Here's how the part is built. I have some questions about the finished solid (model axes, mm). Face numbers are marked on the shaded views. A direction names the side the tool comes from. Round coordinates to 2 decimals unless told otherwise and drop trailing zeros. Loops run counter-clockwise (first coordinate to the right, second up) from the corner with the lowest first, then second, coordinate; pieces in that order, holes last. Notation, with made-up numbers: M 42,-23 L 53,-23 A23 ccw 53,5 Z; hole C 38,-6 d5. An arc over 180 degrees is marked long. Write each question's results on one line, items separated by ' | '. Start each with the question number.
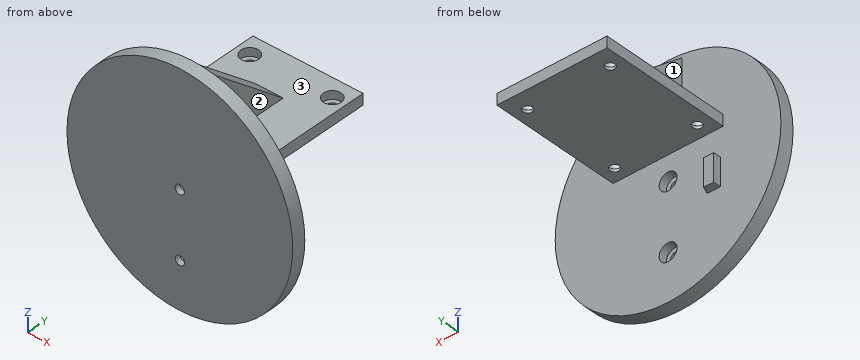
```python
from build123d import *

# Parameters (mm, degrees)
SKETCH1_R                                    = 41
BOSS_EXTRUDE1_DEPTH                          = 5
BOSS_EXTRUDE2_DEPTH                          = 5.08
BOSS_EXTRUDE2_DEPTH_BACK                     = 5.08
SKETCH7_W                                    = 40
SKETCH7_H                                    = 48
BOSS_EXTRUDE3_DEPTH                          = 4
CBORE_FOR_M5_HEX_HEAD_CAP_SCREW5_D           = 3.4
CBORE_FOR_M5_HEX_HEAD_CAP_SCREW5_DEPTH       = 5.5
CBORE_FOR_M5_HEX_HEAD_CAP_SCREW5_CBORE_D     = 6.5
CBORE_FOR_M5_HEX_HEAD_CAP_SCREW5_CBORE_DEPTH = 3
CBORE_FOR_M5_HEX_HEAD_CAP_SCREW5_TIP         = 1.021463052
SKETCH22_W                                   = 4
SKETCH22_H                                   = 10
BOSS_EXTRUDE4_DEPTH                          = 2
BOSS_EXTRUDE5_DEPTH                          = 10
CBORE_FOR_M5_HEX_HEAD_CAP_SCREW6_D           = 3.4
CBORE_FOR_M5_HEX_HEAD_CAP_SCREW6_DEPTH       = 5.5
CBORE_FOR_M5_HEX_HEAD_CAP_SCREW6_CBORE_D     = 6.5
CBORE_FOR_M5_HEX_HEAD_CAP_SCREW6_CBORE_DEPTH = 3
CBORE_FOR_M5_HEX_HEAD_CAP_SCREW6_TIP         = 1.021463052


with BuildPart() as part:
    # Sketch1 → Boss-Extrude1 (new body)
    with BuildSketch(Plane(origin=(0, 0, 0), x_dir=(1, 0, 0), z_dir=(0, 1, 0))):
        with Locations(Location((0, 0, 0), (0, 0, 270))):
            Circle(SKETCH1_R)
    extrude(amount=BOSS_EXTRUDE1_DEPTH)

    # Sketch6 → Boss-Extrude2 (add, two sides: drawn at the far end of the back side and taken through both)
    with BuildSketch(Plane(origin=(0, 0, 0), x_dir=(0, 0, -1), z_dir=(1, 0, 0)).offset(-BOSS_EXTRUDE2_DEPTH_BACK)):
        Polygon((-13, 5), (-39.5, 5), (-13, 37), align=None)
    extrude(amount=BOSS_EXTRUDE2_DEPTH + BOSS_EXTRUDE2_DEPTH_BACK)

    # Sketch7 → Boss-Extrude3 (add)
    with BuildSketch(Plane(origin=(0, 0, 13), x_dir=(-1, 0, 0), z_dir=(0, 0, -1))):
        with Locations((0, 29)):
            Rectangle(SKETCH7_W, SKETCH7_H)
    extrude(amount=BOSS_EXTRUDE3_DEPTH)

    # CBORE for M5 Hex Head Cap Screw5
    with Locations(Plane(origin=(0, 5, 0), x_dir=(1, 0, 0), z_dir=(0, 1, 0))):
        with Locations((0, 0), (0, 24)):
            CounterBoreHole(CBORE_FOR_M5_HEX_HEAD_CAP_SCREW5_D / 2, CBORE_FOR_M5_HEX_HEAD_CAP_SCREW5_CBORE_D / 2, CBORE_FOR_M5_HEX_HEAD_CAP_SCREW5_CBORE_DEPTH, depth=CBORE_FOR_M5_HEX_HEAD_CAP_SCREW5_DEPTH)
            with Locations((0, 0, -(CBORE_FOR_M5_HEX_HEAD_CAP_SCREW5_DEPTH + CBORE_FOR_M5_HEX_HEAD_CAP_SCREW5_TIP / 2))):  # 118° drill point
                Cone(0, CBORE_FOR_M5_HEX_HEAD_CAP_SCREW5_D / 2, CBORE_FOR_M5_HEX_HEAD_CAP_SCREW5_TIP, mode=Mode.SUBTRACT)

    # Sketch22 → Boss-Extrude4 (add)
    with BuildSketch(Plane(origin=(0, 5, 0), x_dir=(1, 0, 0), z_dir=(0, 1, 0))):
        with Locations((-17, 6)):
            Rectangle(SKETCH22_W, SKETCH22_H)
    extrude(amount=BOSS_EXTRUDE4_DEPTH)

    # Sketch23 → Boss-Extrude5 (add)
    with BuildSketch(Plane(origin=(0, 0, -11), x_dir=(-1, 0, 0), z_dir=(0, 0, -1))):
        Polygon((14.171572875, 5), (15.33137085, 7.8), (19, 7.8), (19, 5), align=None)
    extrude(amount=-BOSS_EXTRUDE5_DEPTH)

    # CBORE for M5 Hex Head Cap Screw6
    with Locations(Plane.XY.offset(13)):
        with Locations((15, 10), (-15, 10), (-15, 46), (15, 46)):
            CounterBoreHole(CBORE_FOR_M5_HEX_HEAD_CAP_SCREW6_D / 2, CBORE_FOR_M5_HEX_HEAD_CAP_SCREW6_CBORE_D / 2, CBORE_FOR_M5_HEX_HEAD_CAP_SCREW6_CBORE_DEPTH, depth=CBORE_FOR_M5_HEX_HEAD_CAP_SCREW6_DEPTH)
            with Locations((0, 0, -(CBORE_FOR_M5_HEX_HEAD_CAP_SCREW6_DEPTH + CBORE_FOR_M5_HEX_HEAD_CAP_SCREW6_TIP / 2))):  # 118° drill point
                Cone(0, CBORE_FOR_M5_HEX_HEAD_CAP_SCREW6_D / 2, CBORE_FOR_M5_HEX_HEAD_CAP_SCREW6_TIP, mode=Mode.SUBTRACT)


solid = part.part
```
1. I want a section at D-D on y = 24. List the corners of the cut face in (x, z) for me.
2. I need wall thicknesses on line 1 along Y through (x, z) = (15, 9.4); line 2 along Y through (x, z) = (-15, 11); line 3 along Y through (x, z) = (-6, 35.5). Which ranges of each line are inside material? Lowest first, please.
3. I want a section at C-C on z = -24. List the corners of the cut face in (x, y) for me.
4. I want a section at A-A on x = 0. List the corners of the cut face in (y, z) for me, plus the area to 3 significant figures.
5. For pin 1 (2 mm diameter, centred on x = -8, y = 18.5, fed in from -Z); pin 2 (8.5 mm diameter, centred on x = 15, y = 46, fed in from +Z); pin 3 (2 mm diameter, centred on x = -15.5, y = 7, fed in from -Z); pin 4 (1 mm diameter, centred on x = 12.5, z = -30.5, fed in from -Y), each with a flat end and sliding along its axis, tell me the tip position at first contact or that it passes through.
6. I want a section at B-B on y = 46. List the corners of the cut face in (x, z) for me.
7. Which directions (+Z, -Z, +X, -X, +Y, -Y) give clear straight access to the entire face, cutting with the end or side of a thin tool? Please do the marked faces 1, 2 and 3.
Outcome:
1) outline: M -20,9 L 20,9 L 20,13 L 5.08,13 L 5.08,23.77 L -5.08,23.77 L -5.08,13 L -20,13 Z
2) line 1: 0 to 8.3, 11.7 to 44.3, 47.7 to 53 | line 2: 0 to 6.75, 13.25 to 42.75, 49.25 to 53 | line 3: 0 to 5
3) outline: M -33.24,0 L -1.7,0 L -1.7,2 L -3.25,2 L -3.25,5 L -33.24,5 Z; M 1.7,0 L 33.24,0 L 33.24,5 L 3.25,5 L 3.25,2 L 1.7,2 Z
4) outline: M 0,-41 L 5,-41 L 5,-27.25 L 2,-27.25 L 2,-25.7 L 0,-25.7 Z; M 0,-22.3 L 2,-22.3 L 2,-20.75 L 5,-20.75 L 5,-3.25 L 2,-3.25 L 2,-1.7 L 0,-1.7 Z; M 0,1.7 L 2,1.7 L 2,3.25 L 5,3.25 L 5,9 L 53,9 L 53,13 L 37,13 L 5,39.5 L 5,41 L 0,41 Z | area: 973 mm2
5) pin 1: z = 9 | pin 2: z = 13 | pin 3: z = -11 | pin 4: y = 0
6) outline: M -20,9 L -16.7,9 L -16.7,10 L -18.25,10 L -18.25,13 L -20,13 Z; M -13.3,9 L 13.3,9 L 13.3,10 L 11.75,10 L 11.75,13 L -11.75,13 L -11.75,10 L -13.3,10 Z; M 16.7,9 L 20,9 L 20,13 L 18.25,13 L 18.25,10 L 16.7,10 Z
7) face 1: +Z, -X, +Y | face 2: +Z, +X, +Y | face 3: +Z, +Y
